Autodesk Inventor part; units mm, degrees
ref_plane "YZ Plane" through (0, 0, 0) normal (1, 0, 0) x (0, 1, 0)
ref_plane "XZ Plane" through (0, 0, 0) normal (0, 1, 0) x (-1, 0, 0)
ref_plane "XY Plane" through (0, 0, 0) normal (0, 0, 1) x (1, 0, 0)
sketch "Sketch1" plane through (0, 0, 0) normal (0, 1, 0) x (-1, 0, 0)
  line L0 (38.1, 38.1) -> (-38.1, 38.1)
  line L1 (-38.1, 38.1) -> (-38.1, -38.1)
  line L2 (-38.1, -38.1) -> (38.1, -38.1)
  line L3 (38.1, -38.1) -> (38.1, 38.1)
  line L4 (38.1, 38.1) -> (-38.1, -38.1) construction
  line L5 (-38.1, 38.1) -> (38.1, -38.1) construction
  point P0 (0, 0)
  dimension "d0" = 76.2
  dimension "d1" = 76.2
extrude "Extrusion1" add sketch "Sketch1" along normal blind 101.6
sketch "Sketch2" plane through (38.1, 0, 38.1) normal (1, 0, 0) x (0, 0, -1)
  line L0 (31.7497, 12.5069) -> (76.1457, 101.4069)
  line L1 (76.1457, 101.4069) -> (165.0457, 101.4069) construction
  line L2 (76.1457, 12.5069) -> (31.7497, 12.5069)
  line L3 (76.1457, 12.5069) -> (78.6857, 12.5069)
  line L4 (78.6857, 12.5069) -> (78.6857, 101.4069)
  line L5 (78.6857, 101.4069) -> (76.1457, 101.4069)
  point P0 (38.1, 0)
  dimension "d8" = 88.9
  dimension "d10" = 2.54
  dimension "d11" = 88.9
extrude "Extrusion2" cut sketch "Sketch2" against normal blind 101.6
fillet "Fillet1" radius 25.4 1 edges at (0, 12.5069, 6.3503)
sketch "Sketch3" plane through (38.1, 0, 38.1) normal (1, 0, 0) x (0, 0, -1)
  line L0 (7.62, 25.4) -> (0, 25.4)
  line L1 (26.67, 12.7) -> (7.62, 12.7)
  line L2 (26.67, 12.7) -> (71.066, 101.6)
  line L3 (76.2, 101.6) -> (0, 101.6)
  line L4 (0, 25.4) -> (-2.0413, 103.693)
  line L5 (-2.0413, 103.693) -> (71.066, 101.6)
  line L6 (7.62, 12.7) -> (7.62, 25.4)
  line L7 (50.1015, 49.2551) -> (76.1457, 101.4069)
  point P0 (38.1, 0)
  dimension "d15" = 7.62
  dimension "d17" = 19.05
extrude "Extrusion3" cut sketch "Sketch3" against normal blind 101.6
sketch "Sketch4" plane through (0, 0, 0) normal (0, -1, 0) x (1, 0, 0)
  line L0 (50.8, 45.6457) -> (25.4, 45.6457)
  line L1 (25.4, 45.6457) -> (25.4, -45.6457)
  line L2 (25.4, -45.6457) -> (50.8, -45.6457)
  line L3 (50.8, -45.6457) -> (50.8, 45.6457)
  line L4 (38.1, -32.966) -> (38.1, 11.43)
  line L5 (50.8, 45.6457) -> (25.4, -45.6457) construction
  line L6 (25.4, 45.6457) -> (50.8, -45.6457) construction
  point P0 (0, 0)
  point P1 (38.1, 0)
  dimension "d21" = 25.4
extrude "Extrusion4" cut sketch "Sketch4" against normal blind 101.6
properties part number "hahahaurwelcome"
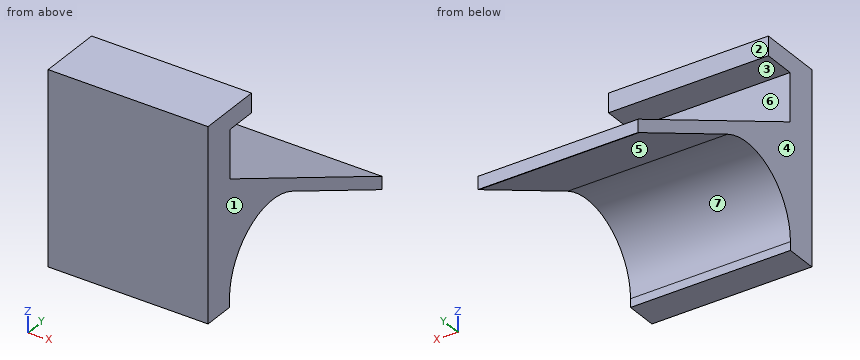
Read the model definition and answer for the solid it produces. Units are mm, in the model's axes. Face numbers are marked on the shaded views. A direction names the side the tool comes from. Give positions to 0.01 mm unless a question says otherwise; leave off trailing zeros. Loops run counter-clockwise (first coordinate to the right, second up) from the corner with the lowest first, then second, coordinate; pieces in that order, holes last. Notation, with made-up numbers: (84.5, 82) -> (102.5, 82) arc R34 ccw to (102.5, 120) -> close; hole circle Ø5 at (31, -31). An arc over 180 degrees is marked (long way). Use a Markdown table: item, result.
Q1. Determine the mould class of the marked faces 4, 5, 6 and 7 for opening direction Y: pulls with the +Y half, pulls with the -Y half, needs draft (parallel to the pull), parting line crosses it, or undercut.
Solved:
| item | result |
|---|---|
| face 4 | needs draft |
| face 5 | undercut |
| face 6 | pulls with the +Y half |
| face 7 | undercut |
Q2. Section D-D, the plane z = 17 is taken. Determine the outline of the cut face in (x, y), then the cut area to 3 significant figures.
Solved:
| item | result |
|---|---|
| outline | (-38.1, 0) -> (25.4, 0) -> (25.4, 12.7) -> (-38.1, 12.7) -> close |
| area | 806 mm^2 |
Q3. Section C-C, the plane x = -34 is taken. Determine the outline of the cut face in (y, z).
Solved:
| item | result |
|---|---|
| outline | (0, -38.1) -> (12.51, -38.1) -> (12.51, -34.73) arc R25.4 cw to (49.26, -12) -> (101.41, -38.05) -> (101.41, -38.1) -> (101.6, -38.1) -> (101.6, -32.97) -> (12.7, 11.43) -> (12.7, 30.48) -> (25.4, 30.48) -> (25.4, 38.1) -> (0, 38.1) -> close |
Q4. Each of these flat-tipped pins is pushed along its axis until it touches: pin 1 (6 mm diameter, centred on x = -9.5, z = -2.5, fed in from +Y); pin 2 (8.5 mm diameter, centred on x = 7, z = 34, fed in from +Y); pin 3 (4 mm diameter, centred on x = -19, y = 37, fed in from -Z). Where does it stop, or does it pass through?
Solved:
| item | result |
|---|---|
| pin 1 | stops at y = 46.6 |
| pin 2 | stops at y = 25.4 |
| pin 3 | stops at z = -9.49 |
Q5. A tool of negligible diameter and unlimited length cuts with its end or side. For the marked faces 1, 2 and 3, from which of +Z, -Z, +X, -X, +Y, -Y can it reach the whole face along a straight path? Write none if from no direction.
Solved:
| item | result |
|---|---|
| face 1 | +Z, -Z, +X, +Y, -Y |
| face 2 | +Z, +X, -X, +Y |
| face 3 | +X, -X, +Y |
Q6. Section A-A, the plane z = -20 is taken. Determine the outline of the cut face in (x, y), then the cut area to 3 significant figures.
Solved:
| item | result |
|---|---|
| outline | (-38.1, 0) -> (25.4, 0) -> (25.4, 17.21) -> (-38.1, 17.21) -> close; (-38.1, 65.27) -> (25.4, 65.27) -> (25.4, 75.64) -> (-38.1, 75.64) -> close |
| area | 1,750 mm^2 |
Q7. Find the intervals of material crossed by line 1 along Y through (x, z) = (-22, 17); line 2 along Y through (x, z) = (6, -14.5); line 3 along Y through (x, z) = (-16.5, -19.5), in increasing order.
Solved:
| item | result |
|---|---|
| line 1 | y = 0 to 12.7 |
| line 2 | y = 0 to 22.54, 54.26 to 64.62 |
| line 3 | y = 0 to 17.58, 64.27 to 74.64 |
Q8. Section B-B, the plane y = 21.5 is taken. Determine the outline of the cut face in (x, z).
Solved:
| item | result |
|---|---|
| outline | (-38.1, -15.34) -> (25.4, -15.34) -> (25.4, 7.04) -> (-38.1, 7.04) -> close; (-38.1, 30.48) -> (25.4, 30.48) -> (25.4, 38.1) -> (-38.1, 38.1) -> close |
